```python
from build123d import *

# Parameters (mm, degrees)
SKETCH_1_W          = 200
SKETCH_1_H          = 120
EXTRUDE_1_DEPTH     = 20
SKETCH_2_W          = 160
SKETCH_2_H          = 100
EXTRUDE_2_DEPTH     = 80
SKETCH_3_W          = 144
SKETCH_3_H          = 84
CUT_EXTRUDE_1_DEPTH = 139.115893365
SKETCH_4_R          = 4
CUT_EXTRUDE_2_DEPTH = 154.622914957
SKETCH_5_R          = 12.5
CUT_EXTRUDE_3_DEPTH = 201


with BuildPart() as part:
    # 草图1 → 凸台-拉伸1 (new body)
    with BuildSketch(Plane(origin=(0, 0, 0), x_dir=(1, 0, 0), z_dir=(0, 1, 0))):
        Rectangle(SKETCH_1_W, SKETCH_1_H)
    extrude(amount=EXTRUDE_1_DEPTH)

    # 草图2 → 凸台-拉伸2 (add)
    with BuildSketch(Plane(origin=(0, 20, 0), x_dir=(1, 0, 0), z_dir=(0, 1, 0))):
        Rectangle(SKETCH_2_W, SKETCH_2_H)
    extrude(amount=EXTRUDE_2_DEPTH)

    # 草图3 → 切除-拉伸1 (cut, through all)
    with BuildSketch(Plane(origin=(0, 26, 0), x_dir=(1, 0, 0), z_dir=(0, 1, 0))):
        Rectangle(SKETCH_3_W, SKETCH_3_H)
    extrude(amount=CUT_EXTRUDE_1_DEPTH, mode=Mode.SUBTRACT)

    # 草图4 → 切除-拉伸2 (cut, through all)
    with BuildSketch(Plane(origin=(0, 0, 0), x_dir=(1, 0, 0), z_dir=(0, 1, 0))):
        with Locations(Location((85, -45, 0), (0, 0, 90))):
            Circle(SKETCH_4_R)
        with Locations(Location((85, 45, 0), (0, 0, 90))):
            Circle(SKETCH_4_R)
        with Locations(Location((-85, -45, 0), (0, 0, 90))):
            Circle(SKETCH_4_R)
        with Locations(Location((-85, 45, 0), (0, 0, 90))):
            Circle(SKETCH_4_R)
    extrude(amount=CUT_EXTRUDE_2_DEPTH, mode=Mode.SUBTRACT)

    # 草图5 → 切除-拉伸3 (cut, symmetric)
    with BuildSketch(Plane.XY):
        with Locations((0, 60)):
            Circle(SKETCH_5_R)
    extrude(amount=CUT_EXTRUDE_3_DEPTH, both=True, mode=Mode.SUBTRACT)


solid = part.part
```
For this review, take the finished solid that the model builds, in its own axes (mm). A direction names the side the tool comes from. Coordinates: 2 decimals unless noted, no trailing zeros. Write each loop counter-clockwise with the first axis right and the second up, starting at its lowest first coordinate (ties: lowest second). Pieces come first, ordered by that corner, then holes. Notation, with made-up numbers: (43.5, 32.25) - (71.5, 32.25) arc R21 ccw to (71.5, 38.25) - close; hole circle Ø7 at (6, 84). An arc over 180 degrees is marked (long way). Answer in a Markdown table with one row per item. Add a question column.
Q1. We need section A-A, the plane x = 0. State the section outline as (y, z) points, and give its area (3 significant figures).
Q2. Draft analysis for pull direction X (two halves, no side actions). For faces 4 (the flat face through (-72, 62, 1)), 5 (the cylindrical face through (-81.095, 9.86, -44.133)), 6 (the flat face through (-80, 59, 1)), 7 (the flat face through (100, 10, 1)), state which applies: +X half, -X half, draft (parallel to the pull), parting line (faces both ways), or undercut.
Q3. Tool access review of faces 1 (the flat face through (-17, 62, -42)), 2 (the flat face through (-19, 59, -50)), 3 (the flat face through (-19, 59, 50)): name each direction out of +Z, -Z, +X, -X, +Y, -Y from which nothing blocks a thin tool from reaching the whole face with its end or side.
Q4. We need section B-B, the plane z = 45. State the section outline as (x, y) points.
Q5. We need section C-C, the plane y = 60. State the section outline as (x, z) points, and give its area (3 significant figures).
Q6. We need section D-D, the plane z = -34. State the section outline as (x, y) points, and give its area (3 significant figures).
Q7. For probe 1 along Z at (x, y) = (85, 5); probe 2 along X at (y, z) = (4.5, -45); probe 3 along X at (y, z) = (78.5, -9.5), list the stretches that pass through material, from the lowest coordinate up.
Q8. For P1, Ø1.5, axis at y = 55.5, z = 2, coming from the -X side; P2, Ø10, axis at x = -42.5, y = 56.5, coming from the -Z side; P3, Ø4, axis at x = 67.5, z = -6.5, coming from the +Y side, all flat-tipped, find the tip position at first contact; note any pin that passes through.
Answer list:
| question | item | result |
|---|---|---|
| 1 | outline | (0, -60) - (20, -60) - (20, -50) - (47.5, -50) - (47.5, -42) - (26, -42) - (26, 42) - (47.5, 42) - (47.5, 50) - (20, 50) - (20, 60) - (0, 60) - close; (72.5, -50) - (100, -50) - (100, -42) - (72.5, -42) - close; (72.5, 42) - (100, 42) - (100, 50) - (72.5, 50) - close |
| 1 | area | 3,780 mm2 |
| 2 | face 4 | undercut |
| 2 | face 5 | undercut |
| 2 | face 6 | -X half |
| 2 | face 7 | +X half |
| 3 | face 1 | +Y |
| 3 | face 2 | -Z, +X, -X, +Y |
| 3 | face 3 | +Z, +X, -X, +Y |
| 4 | outline | (-100, 0) - (-89, 0) - (-89, 20) - (-100, 20) - close; (-81, 0) - (81, 0) - (81, 20) - (80, 20) - (80, 100) - (-80, 100) - (-80, 20) - (-81, 20) - close; (89, 0) - (100, 0) - (100, 20) - (89, 20) - close; hole circle Ø25 at (0, 60) |
| 5 | outline | (-80, -50) - (-12.5, -50) - (-12.5, -42) - (-72, -42) - (-72, 42) - (-12.5, 42) - (-12.5, 50) - (-80, 50) - close; (12.5, -50) - (80, -50) - (80, 50) - (12.5, 50) - (12.5, 42) - (72, 42) - (72, -42) - (12.5, -42) - close |
| 5 | area | 3,500 mm2 |
| 6 | outline | (-100, 0) - (100, 0) - (100, 20) - (80, 20) - (80, 100) - (72, 100) - (72, 26) - (-72, 26) - (-72, 100) - (-80, 100) - (-80, 20) - (-100, 20) - close |
| 6 | area | 6,140 mm2 |
| 7 | probe 1 | z = -60 to -49, -41 to 41, 49 to 60 |
| 7 | probe 2 | x = -100 to -89, -81 to 81, 89 to 100 |
| 7 | probe 3 | x = -80 to -72, 72 to 80 |
| 8 | P1 | stops at x = -80 |
| 8 | P2 | stops at z = -50 |
| 8 | P3 | stops at y = 26 |
